Input: dimensioned drawing with shaded views. Units: mm. Origin: part minimum x, y, z. Coordinates: 2 decimals unless noted, no trailing zeros. Order: outer loops, then holes, each group sorted by start corner. A loop starts at its lowest first (then second) coordinate and runs counter-clockwise, first axis right, second up. Notation, with made-up numbers: M 66,3 L 94,3 A26 ccw 94,38 Z; hole C 4.25,47 d4. An arc over 180 degrees is marked long. Write item = value, one per line.
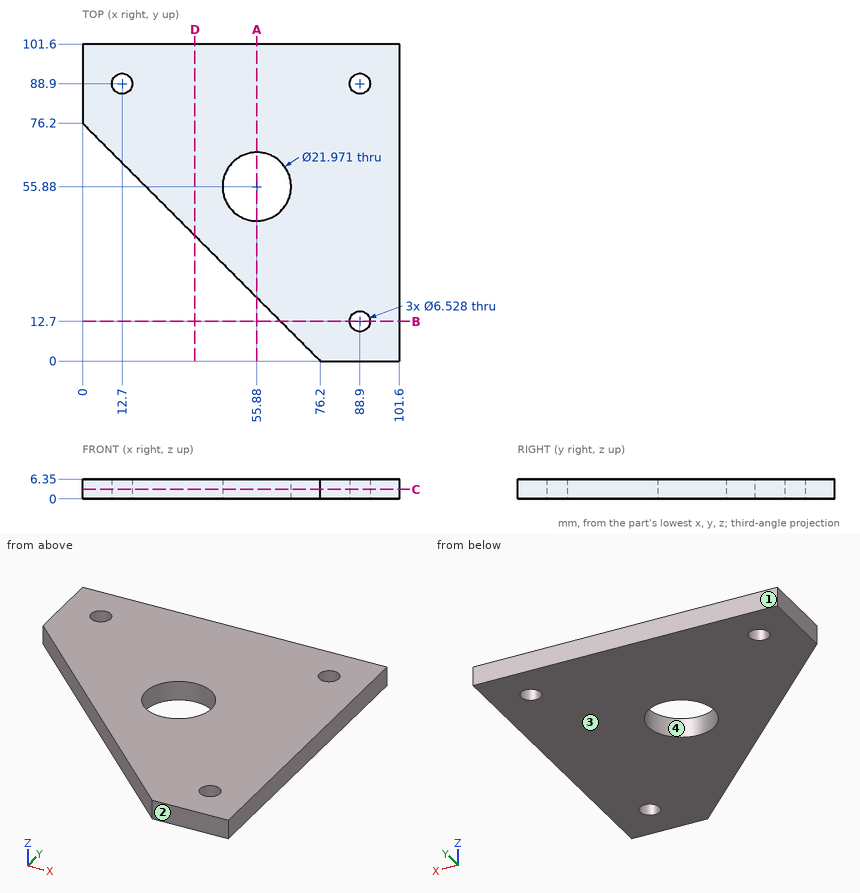
1) Line query: L1, parallel to Y at x = 88.9, z = 1.75; L2, parallel to X at y = 91, z = 3; L3, parallel to X at y = 14, z = 1.5 (1 decimal). Output: solid intervals per line, ascending.
Numbers:
L1 = 0 to 9.44, 15.96 to 85.64, 92.16 to 101.6
L2 = 0 to 10.2, 15.2 to 86.4, 91.4 to 101.6
L3 = 62.2 to 85.9, 91.9 to 101.6
2) Section D-D, the plane x = 36. Return loops of the section in (y, z), and give its area (3 significant figures).
Numbers:
outline = M 40.2,0 L 101.6,0 L 101.6,6.35 L 40.2,6.35 Z
area = 390 mm²
3) Section A-A, the plane x = 55.88. Return loops of the section in (y, z).
Numbers:
outline = M 20.32,0 L 44.89,0 L 44.89,6.35 L 20.32,6.35 Z; M 66.87,0 L 101.6,0 L 101.6,6.35 L 66.87,6.35 Z
4) Mould query, pull axis Y, two halves, no side actions, for the marked faces 1, 2, 3 and 4. Classes: pulls with the +Y half, pulls with the -Y half, needs draft (parallel to the pull), parting line crosses it, or undercut.
Numbers:
face_1 = pulls with the +Y half
face_2 = pulls with the -Y half
face_3 = needs draft
face_4 = undercut
5) Section C-C, the plane z = 3. Return loops of the section in (x, y).
Numbers:
outline = M 0,76.2 L 76.2,0 L 101.6,0 L 101.6,101.6 L 0,101.6 Z; hole C 12.7,88.9 d6.53; hole C 55.88,55.88 d21.97; hole C 88.9,12.7 d6.53; hole C 88.9,88.9 d6.53
6) Section B-B, the plane y = 12.7. Return loops of the section in (x, z).
Numbers:
outline = M 63.5,0 L 85.64,0 L 85.64,6.35 L 63.5,6.35 Z; M 92.16,0 L 101.6,0 L 101.6,6.35 L 92.16,6.35 Z
